Geometry check sheet. Reference: the model listing, model coordinates, mm. Face numbers are marked on the shaded views. A direction names the side the tool comes from. Round coordinates to 2 decimals unless told otherwise and drop trailing zeros. Order: outer loops, then holes, each group sorted by start corner. A loop starts at its lowest first (then second) coordinate and runs counter-clockwise, first axis right, second up. Notation, with made-up numbers: M 40.25,86 L 53.25,86 A28 ccw 53.25,115 Z; hole C -10,47 d4. An arc over 180 degrees is marked long. Return JSON: item names as keys, results as strings. Group by question number.
```python
from build123d import *

# Parameters (mm, degrees)
SKETCH1_R           = 6
BOSS_EXTRUDE1_DEPTH = 5
SKETCH2_R           = 5
BOSS_EXTRUDE2_DEPTH = 4
CUT_EXTRUDE1_DEPTH  = 3
SKETCH4_W           = 2
SKETCH4_H           = 1
CUT_EXTRUDE2_DEPTH  = 10


with BuildPart() as part:
    # Sketch1 → Boss-Extrude1 (new body)
    with BuildSketch(Plane.XY):
        Circle(SKETCH1_R)
    extrude(amount=BOSS_EXTRUDE1_DEPTH)

    # Sketch2 → Boss-Extrude2 (add)
    with BuildSketch(Plane.XY.offset(5)):
        Circle(SKETCH2_R)
    extrude(amount=BOSS_EXTRUDE2_DEPTH)

    # Sketch3 → Cut-Extrude1 (cut)
    with BuildSketch(Plane.XY.offset(9)):
        Polygon((2.048231561, -3.749410728), (4.27120072, -0.1008848), (2.222969159, 3.648525928), (-2.048231561, 3.749410728), (-4.27120072, 0.1008848), (-2.222969159, -3.648525928), align=None)
    extrude(amount=-CUT_EXTRUDE1_DEPTH, mode=Mode.SUBTRACT)

    # Sketch4 → Cut-Extrude2 (cut)
    with BuildSketch(Plane(origin=(0, 0, 0), x_dir=(-1, 0, 0), z_dir=(0, 0, -1))):
        Polygon((5.957011587, -3.709988269), (5.369226334, -4.519005263), (3.751192346, -3.343434759), (4.338977598, -2.534417764), align=None)
        with Locations((6, 0)):
            Rectangle(SKETCH4_W, SKETCH4_H)
        Polygon((2.638647219, -6.502887117), (1.687590702, -6.811904111), (1.069556714, -4.909791079), (2.02061323, -4.600774084), align=None)
        Polygon((-1.687590702, -6.811904111), (-2.638647219, -6.502887117), (-2.02061323, -4.600774084), (-1.069556714, -4.909791079), align=None)
        Polygon((-5.369226334, -4.519005263), (-5.957011587, -3.709988269), (-4.338977598, -2.534417764), (-3.751192346, -3.343434759), align=None)
        with Locations((-6, 0)):
            Rectangle(SKETCH4_W, SKETCH4_H)
        Polygon((-5.957011587, 3.709988269), (-5.369226334, 4.519005263), (-3.751192346, 3.343434759), (-4.338977598, 2.534417764), align=None)
        Polygon((-2.638647219, 6.502887117), (-1.687590702, 6.811904111), (-1.069556714, 4.909791079), (-2.02061323, 4.600774084), align=None)
        Polygon((1.687590702, 6.811904111), (2.638647219, 6.502887117), (2.02061323, 4.600774084), (1.069556714, 4.909791079), align=None)
        Polygon((5.369226334, 4.519005263), (5.957011587, 3.709988269), (4.338977598, 2.534417764), (3.751192346, 3.343434759), align=None)
    extrude(amount=-CUT_EXTRUDE2_DEPTH, mode=Mode.SUBTRACT)


solid = part.part
```
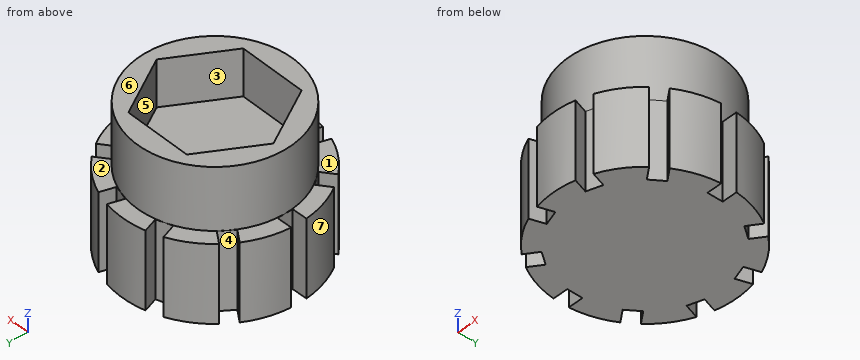
Q1. Material ranges on line 1 along Y through (x, z) = (-4, 2.5); line 2 along Z through (x, y) = (2.5, -1); line 3 along X through (y, z) = (5.25, 1.5), recorded low to high.
Q2. Section check C-C on x = 0. Record the cut outline in (y, z).
Q3. Section check A-A on z = 7.25. Record the cut outline in (x, y).
Q4. Depth check by flat-ended pin: pin 1 Ø3 at (y, z) = (1.5, 7) entering from +X; pin 2 Ø0.6 at (x, y) = (-5.5, 1.5) entering from +Z; pin 3 Ø0.8 at (x, z) = (5.5, 3.5) entering from -Y. Enter the tip coordinate at first touch or a pass-through.
Q5. Section check B-B on y = -1. Record the cut outline in (x, z), plus the area to 3 significant figures.
Q6. Set-up check for the marked faces 1, 2 and 3: record each of +Z, -Z, +X, -X, +Y, -Y from which the full face is reachable in a straight line by a thin tool's end or side.
Q7. Release check for a two-part mould opening along X. For the marked faces 4, 5, 6 and 7 record: +X half, -X half, draft (parallel to the pull), parting line (faces both ways), or undercut.
Geometry check:
{
 "1": {"line 1": "y = -4.47 to -3.52, -3 to 3, 3.52 to 4.47", "line 2": "z = 0 to 6", "line 3": "x = -2.9 to -2.23, -1.18 to 1.18, 2.23 to 2.9"},
 "2": {"outline": "M -6,0 L 6,0 L 6,5 L 5,5 L 5,9 L 3.7,9 L 3.7,6 L -3.7,6 L -3.7,9 L -5,9 L -5,5 L -6,5 Z"},
 "3": {"outline": "C 0,0 d10; hole M -4.27,0.1 L -2.22,-3.65 L 2.05,-3.75 L 4.27,-0.1 L 2.22,3.65 L -2.05,3.75 Z"},
 "4": {"pin 1": "stops at x = 5", "pin 2": "stops at z = 5", "pin 3": "stops at y = -3.11"},
 "5": {"outline": "M -5.92,0 L 5.92,0 L 5.92,5 L 4.9,5 L 4.9,9 L 3.72,9 L 3.72,6 L -3.67,6 L -3.67,9 L -4.9,9 L -4.9,5 L -5.92,5 Z", "area": "76.2 mm^2"},
 "6": {"face 1": "+Z, -X, -Y", "face 2": "+Z, +X, +Y", "face 3": "+Z"},
 "7": {"face 4": "undercut", "face 5": "undercut", "face 6": "draft", "face 7": "-X half"}
}
